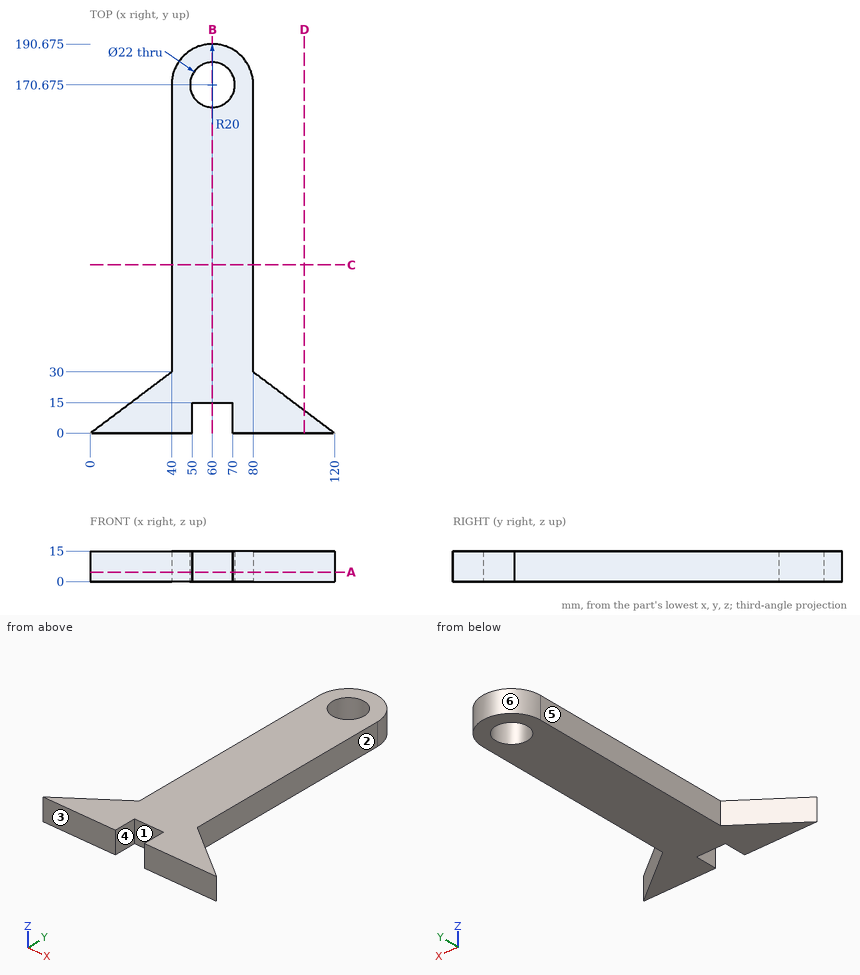
Geometry: see drawing. Coordinates: mm, zero at the bounding-box minimum. A direction names the side the tool comes from. Give positions to 0.01 mm unless a question says otherwise; leave off trailing zeros. Order: outer loops, then holes, each group sorted by start corner. A loop starts at its lowest first (then second) coordinate and runs counter-clockwise, first axis right, second up. Notation, with made-up numbers: (38.25, 76) -> (42.25, 76) arc R19 cw to (42.25, 81) -> close; hole circle Ø6 at (35, 65). An arc over 180 degrees is marked (long way). Write each question's results on one line, items separated by ' | '. Start each with the question number.
1) Line query: line 1 (Y direction, x = 60, z = 7.75) (3 decimals); line 2 (X direction, y = 127, z = 8.5); line 3 (Y direction, x = 38, z = 4). Output: solid intervals per line, ascending. Write a range as from..to.
2) Section B-B (x = 60). Return loops of the section in (y, z) (3 decimals), then the cut area to 3 significant figures.
3) Draft query along X for the marked faces 1, 2 and 3. Return one class per face: pulls with the +X half, pulls with the -X half, needs draft (parallel to the pull), parting line crosses it, or undercut.
4) Section C-C (y = 82.5). Return loops of the section in (x, z).
5) Section A-A (z = 4.75). Return loops of the section in (x, y) (3 decimals).
6) Set-up query: the marked faces 4, 5 and 6. Return all of +Z, -Z, +X, -X, +Y, -Y with unobstructed straight access to the full face (end or side cutting, diameter ignored); none if empty.
7) Section D-D (x = 105). Return loops of the section in (y, z), then the cut area to 3 significant figures.
8) First-contact query: pin 1 (2 mm diameter, centred on y = 30, z = 7.5, fed in from -X); pin 2 (4 mm diameter, centred on y = 140, z = 9, fed in from +X); pin 3 (4 mm diameter, centred on y = 38.5, z = 5.5, fed in from -X). Flat tips, straight axial feed; report the tip coordinate or a pass-through.
Calculated:
1) line 1: 15..159.675, 181.675..190.675 | line 2: 40..80 | line 3: 0..28.5
2) outline: (15, 0) -> (159.675, 0) -> (159.675, 15) -> (15, 15) -> close; (181.675, 0) -> (190.675, 0) -> (190.675, 15) -> (181.675, 15) -> close | area: 2,310 mm2
3) face 1: undercut | face 2: pulls with the +X half | face 3: needs draft
4) outline: (40, 0) -> (80, 0) -> (80, 15) -> (40, 15) -> close
5) outline: (0, 0) -> (50, 0) -> (50, 15) -> (70, 15) -> (70, 0) -> (120, 0) -> (80, 30) -> (80, 170.675) arc R20 ccw to (40, 170.675) -> (40, 30) -> close; hole circle Ø22 at (60, 170.675)
6) face 4: +Z, -Z, -Y | face 5: +Z, -Z, -X, +Y | face 6: +Z, -Z, +Y
7) outline: (0, 0) -> (11.25, 0) -> (11.25, 15) -> (0, 15) -> close | area: 169 mm2
8) pin 1: x = 38.67 | pin 2: x = 80 | pin 3: x = 40
